The model under review builds one solid part; all positions refer to its coordinate system, in mm. A direction names the side the tool comes from. Coordinates: 2 decimals unless noted, no trailing zeros. Loops run counter-clockwise (first coordinate to the right, second up) from the corner with the lowest first, then second, coordinate; pieces in that order, holes last. Notation, with made-up numbers: (60.5, 54.5) - (65.5, 54.5) arc R37 cw to (65.5, 92.5) - close; hole circle Ø5 at (79, -7). An arc over 180 degrees is marked (long way). Use a Markdown table: item, result. Add a question column.
1) Add section A-A, the plane z = 0. Give the boundary of the cut face in (x, y), and give its area (3 significant figures).
2) For faces 4 (the flat face through (-10.1, 2, -24.3)), 5 (the flat face through (-14, 6, -21)), 6 (the flat face through (-10.1, 0, -24.3)), list the 3-axis set-ups (+Z, -Z, +X, -X, +Y, -Y) from which the entire face can be reached by the end or side of a thin tool; tool diameter is ignored.
3) Add section B-B, the plane x = 0. Give the boundary of the cut face in (y, z).
4) To check wall thickness, follow L1, parallel to Z at x = 0, y = 2.5; L2, parallel to Z at x = 0, y = 0.5. State the ranges of each line that lie inside material, in increasing order. Write a range as [from, to].
5) The part is to be moulded in two halves that separate along Z. For faces 1 (the cylindrical face through (-20.633, 3.972, -15.821)), 2 (the cylindrical face through (23.846, 0.93, 7.509)), 3 (the flat face through (-14, -4, 21)), say which applies: pulls with the +Z half, pulls with the -Z half, needs draft (parallel to the pull), parting line crosses it, or undercut.
6) Add section C-C, the plane y = 4.5. Give the boundary of the cut face in (x, z), and give its area (3 significant figures).
7) Clearance check with flat-ended pins moving along their axes: pin 1 (1.5 mm diameter, centred on y = -2.5, z = 15, fed in from -X); pin 2 (6 mm diameter, centred on y = -0.5, z = 20, fed in from -X); pin 3 (3 mm diameter, centred on y = -1, z = 15, fed in from +X). State where each tip first meets the part, or that it passes through.
Autodesk Inventor part; units mm, degrees
ref_plane "YZ Plane" through (0, 0, 0) normal (1, 0, 0) x (0, 1, 0)
ref_plane "XZ Plane" through (0, 0, 0) normal (0, 1, 0) x (-1, 0, 0)
ref_plane "XY Plane" through (0, 0, 0) normal (0, 0, 1) x (1, 0, 0)
sketch "Sketch5" plane through (0, 0, 0) normal (0, 1, 0) x (-1, 0, 0)
  circle A0 centre (0, 0) radius 27.5
  dimension "d18" = 55
extrude "Extrusion5" add sketch "Sketch5" along normal blind 2
sketch "Sketch6" plane through (0, 2, 0) normal (0, 1, 0) x (1, 0, 0)
  circle A0 centre (0, 0) radius 26
  dimension "d21" = 52
extrude "Extrusion6" add sketch "Sketch6" along normal blind 4
sketch "Sketch7" plane through (0, 6, 0) normal (0, 1, 0) x (1, 0, 0)
  circle A0 centre (0, 0) radius 25
  dimension "d24" = 50
extrude "Extrusion7" cut sketch "Sketch7" against normal through all
thread "Thread4"
sketch "Sketch8" plane through (0, 0, 0) normal (0, -1, 0) x (1, 0, 0)
  circle A0 centre (0, 0) radius 26
  dimension "d29" = 52
extrude "Extrusion8" add sketch "Sketch8" along normal blind 4
sketch "Sketch9" plane through (0, -4, 0) normal (0, -1, 0) x (1, 0, 0)
  circle A0 centre (0, 0) radius 25
  dimension "d32" = 50
extrude "Extrusion9" cut sketch "Sketch9" against normal blind 4
thread "Thread5"
properties part number "77mm to 52mm" material "Aluminum 6061-AHC"
From the geometry:
| question | item | result |
|---|---|---|
| 1 | outline | (-27.5, 0) - (-26, 0) - (-26, -4) - (-25, -4) - (-25, 6) - (-26, 6) - (-26, 2) - (-27.5, 2) - close; (25, -4) - (26, -4) - (26, 0) - (27.5, 0) - (27.5, 2) - (26, 2) - (26, 6) - (25, 6) - close |
| 1 | area | 26.0 mm^2 |
| 2 | face 4 | +Y |
| 2 | face 5 | +Z, -Z, +X, -X, +Y |
| 2 | face 6 | -Y |
| 3 | outline | (-4, -26) - (0, -26) - (0, -27.5) - (2, -27.5) - (2, -26) - (6, -26) - (6, -25) - (-4, -25) - close; (-4, 25) - (6, 25) - (6, 26) - (2, 26) - (2, 27.5) - (0, 27.5) - (0, 26) - (-4, 26) - close |
| 4 | L1 | z = [-26, -25], [25, 26] |
| 4 | L2 | z = [-27.5, -25], [25, 27.5] |
| 5 | face 1 | parting line crosses it |
| 5 | face 2 | undercut |
| 5 | face 3 | needs draft |
| 6 | outline | circle Ø52 at (0, 0); hole circle Ø50 at (0, 0) |
| 6 | area | 160 mm^2 |
| 7 | pin 1 | stops at x = -21.75 |
| 7 | pin 2 | stops at x = -21.58 |
| 7 | pin 3 | stops at x = 23.74 |
